Solid Edge part; units mm, degrees
sketch "Sketch1" plane through (0, 0, 0) normal (0, 0, 1) x (1, 0, 0)
  line L0 (35, 0) -> (35, 30)
  line L1 (35, 30) -> (0, 30)
  line L2 (-35, 30) -> (0, 30)
  line L3 (-35, 0) -> (-35, 30)
  line L4 (-10, 0) -> (-35, 0)
  line L5 (-10, 10) -> (-10, 0)
  line L6 (-20, 10) -> (-10, 10)
  line L7 (-20, 20) -> (-20, 10)
  line L8 (0, 20) -> (-20, 20)
  line L9 (0, 20) -> (20, 20)
  line L10 (20, 20) -> (20, 10)
  line L11 (20, 10) -> (10, 10)
  line L12 (10, 10) -> (10, 0)
  line L13 (10, 0) -> (35, 0)
extrude "Protrusion1" add sketch "Sketch1" along normal mid plane 180
sketch "Sketch2" plane through (35, 15, 0) normal (1, 0, 0) x (0, 0, -1)
  line L0 (-70, 15) -> (-70, 33)
  line L1 (-70, 15) -> (-30, 15)
  line L2 (-30, 15) -> (-30, 55)
  line L3 (-30, 55) -> (-48, 55)
  arc A0 (-48, 55) -> (-70, 33) centre (-70, 55) cw
  line L4 (60, 15) -> (60, 35)
  line L5 (60, 35) -> (90, 35)
  line L6 (90, 35) -> (90, 15)
  line L7 (90, 15) -> (60, 15)
extrude "ExtrudedProtrusion_4" add sketch "Sketch2" against normal blind 70
sketch "Sketch3" plane through (0, 25, -90) normal (0, 0, -1) x (-1, 0, 0)
  circle A0 centre (0, 25) radius 10
extrude "ExtrudedCutout_3" cut sketch "Sketch3" against normal blind 30
sketch "Sketch4" plane through (0, 25, -90) normal (0, 0, -1) x (-1, 0, 0)
  line L0 (10, 25) -> (35, 25)
  line L1 (-35, 25) -> (-10, 25)
  arc A0 (-35, 25) -> (35, 25) centre (0, 25) cw
  arc A1 (-10, 25) -> (10, 25) centre (0, 25) cw
extrude "ExtrudedProtrusion_5" add sketch "Sketch4" against normal blind 30
sketch "Sketch5" plane through (0, 30, -15) normal (0, 1, 0) x (-1, 0, 0)
  circle A0 centre (0, -35) radius 10
extrude "ExtrudedCutout_4" cut sketch "Sketch5" against normal blind 30
Build history of the part. All positions in model axes, mm. A direction names the side the tool comes from. Give positions to 0.01 mm unless a question says otherwise; leave off trailing zeros. Write each loop counter-clockwise with the first axis right and the second up, starting at its lowest first coordinate (ties: lowest second). Pieces come first, ordered by that corner, then holes. Notation, with made-up numbers: (33.5, 56) - (52.5, 56) arc R18 cw to (52.5, 85) - close; hole circle Ø4 at (0, 76). An arc over 180 degrees is marked (long way). Use one line per item in the form item = value. Start each with the question number.
1. Band-saw the part on C-C on y = 52. Write the cut outline in (x, z).
2. 3-axis set-ups, long thin cutter, end or side, ignore diameter. For faces 1 (the face through (0, 30, -16)), 2 (the face through (0, 20, -1)), 3 (the face through (0, 39, 70)), 4 (the face through (-10, 5, -1)): which of +Z, -Z, +X, -X, +Y, -Y reach the whole face in a straight line?
3. Probe line 1 (Z direction, x = 0, y = 27); line 2 (X direction, y = 8.5, z = 68.5); line 3 (Z direction, x = 13.5, y = 37). List the from-to ranges inside material, lowest first. Write a range as [from, to].
4. Band-saw the part on A-A on z = -50. Write the cut outline in (x, y), plus the area to 3 significant figures.
5. Band-saw the part on B-B on x = -18. Write the cut outline in (y, z).
6. Drop flat-ended pins along their axis: pin 1 Ø14.5 at (x, y) = (-6.5, 42.5) entering from +Z; pin 2 Ø4 at (x, z) = (0, -59.5) entering from -Y; pin 3 Ø20 at (x, z) = (-14, 35.5) entering from +Y. Give the stop position or say it passes through.
7. Two-plate mould, pull along X, no slides. Class faces 5 (the face through (0, 50, 30)), 6 (the face through (2.17, 25.07, -59.76)), 7 (the face through (2.17, 40.24, -75.21)), 8 (the face through (-0.77, 84.99, -75.21)): released by +X, released by -X, zero draft, split by the parting line, or undercut.
8. Band-saw the part on D-D on x = 28. Write the cut outline in (y, z).
Conclusion:
q1.outline = (-35, 30) - (35, 30) - (35, 57.35) - (-35, 57.35) - close; (-34.94, -90) - (-9.8, -90) - (-9.8, -60) - (-34.94, -60) - close; (9.8, -90) - (34.94, -90) - (34.94, -60) - (9.8, -60) - close
q2.face_1 = +X, -X, +Y
q2.face_2 = +Z, -Z
q2.face_3 = +Z, +X, -X, +Y
q2.face_4 = +Z, -Z, -Y
q3.line_1 = [-90, -60], [-40, 90]
q3.line_2 = [-35, -10], [10, 35]
q3.line_3 = [-90, -60], [30, 70]
q4.outline = (-35, 0) - (-10, 0) - (-10, 10) - (-20, 10) - (-20, 20) - (-10, 20) - (-10, 30) - (-35, 30) - close; (10, 0) - (35, 0) - (35, 30) - (10, 30) - (10, 20) - (20, 20) - (20, 10) - (10, 10) - close
q4.area = 1,300 mm²
q5.outline = (0, -90) - (10, -90) - (10, 90) - (0, 90) - close; (20, -90) - (80.02, -90) - (80.02, -60) - (30, -60) - (30, 30) - (70, 30) - (70, 48) arc R22 cw to (48, 70) - (30, 70) - (30, 90) - (20, 90) - close
q6.pin_1 = 70
q6.pin_2 = 20
q6.pin_3 = 70
q7.face_5 = zero draft
q7.face_6 = undercut
q7.face_7 = undercut
q7.face_8 = split by the parting line
q8.outline = (0, -90) - (71, -90) - (71, -60) - (30, -60) - (30, 30) - (70, 30) - (70, 48) arc R22 cw to (48, 70) - (30, 70) - (30, 90) - (0, 90) - close
